Check sheet for the modelled part. Datum: model origin and axes. Units: mm. A direction names the side the tool comes from. Round coordinates to 2 decimals unless told otherwise and drop trailing zeros. Order: outer loops, then holes, each group sorted by start corner. A loop starts at its lowest first (then second) coordinate and runs counter-clockwise, first axis right, second up. Notation, with made-up numbers: (-1.75, 6) -> (52.25, 6) arc R18 ccw to (52.25, 38) -> close; hole circle Ø11 at (52, 8.5). An arc over 180 degrees is marked (long way). Answer in a Markdown table with one row per item.
from build123d import *

# Parameters (mm, degrees)
SKETCH1_R           = 4
SKETCH1_R_2         = 1.5
BOSS_EXTRUDE1_DEPTH = 4
SKETCH2_R           = 3.5
SKETCH2_R_2         = 2
CUT_EXTRUDE1_DEPTH  = 0.2
CUT_EXTRUDE2_START  = -0.2
SKETCH3_R           = 3.5
SKETCH3_R_2         = 2
CUT_EXTRUDE2_DEPTH  = 0.2


with BuildPart() as part:
    # Sketch1 → Boss-Extrude1 (new body)
    with BuildSketch(Plane(origin=(0, 0, 0), x_dir=(0, 0, -1), z_dir=(1, 0, 0))):
        Circle(SKETCH1_R)
        Circle(SKETCH1_R_2, mode=Mode.SUBTRACT)
    extrude(amount=BOSS_EXTRUDE1_DEPTH)

    # Sketch2 → Cut-Extrude1 (cut)
    with BuildSketch(Plane(origin=(4, 0, 0), x_dir=(0, 0, -1), z_dir=(1, 0, 0))):
        Circle(SKETCH2_R)
        Circle(SKETCH2_R_2, mode=Mode.SUBTRACT)
    extrude(amount=-CUT_EXTRUDE1_DEPTH, mode=Mode.SUBTRACT)

    # Sketch3 → Cut-Extrude2 (cut)
    with BuildSketch(Plane.ZY.offset(CUT_EXTRUDE2_START)):
        with Locations(Location((0, 0, 0), (0, 0, 180))):
            Circle(SKETCH3_R)
        with Locations(Location((0, 0, 0), (0, 0, 180))):
            Circle(SKETCH3_R_2, mode=Mode.SUBTRACT)
    extrude(amount=CUT_EXTRUDE2_DEPTH, mode=Mode.SUBTRACT)


solid = part.part
Item 1: Cross-section at D-D (x = 0.4). Record the boundary of the cut face in (y, z), and give its area (3 significant figures).
Result sheet:
| item | result |
|---|---|
| outline | circle Ø8 at (0, 0); hole circle Ø3 at (0, 0) |
| area | 43.2 mm^2 |
Item 2: Depth check by flat-ended pin: P1, Ø1.5, axis at x = 3, y = 1.5, coming from the +Z side; P2, Ø2, axis at x = 3.5, y = -2, coming from the -Z side; P3, Ø1.5, axis at x = 3.5, z = 2, coming from the +Y side. Enter the tip coordinate at first touch or a pass-through.
Result sheet:
| item | result |
|---|---|
| P1 | stops at z = 3.93 |
| P2 | stops at z = -3.87 |
| P3 | stops at y = 3.8 |
Item 3: Mould release check, pull along Y, two halves, no side actions. Record for faces 3 (the flat face through (3.8, -2, -2)), 4 (the cylindrical face through (1.972, -3.905, 0.867)): pulls with the +Y half, pulls with the -Y half, needs draft (parallel to the pull), parting line crosses it, or undercut.
Result sheet:
| item | result |
|---|---|
| face 3 | undercut |
| face 4 | parting line crosses it |
Item 4: Cross-section at A-A (z = 0). Record the boundary of the cut face in (x, y).
Result sheet:
| item | result |
|---|---|
| outline | (0, -4) -> (4, -4) -> (4, -3.5) -> (3.8, -3.5) -> (3.8, -2) -> (4, -2) -> (4, -1.5) -> (0, -1.5) -> (0, -2) -> (0.2, -2) -> (0.2, -3.5) -> (0, -3.5) -> close; (0, 1.5) -> (4, 1.5) -> (4, 2) -> (3.8, 2) -> (3.8, 3.5) -> (4, 3.5) -> (4, 4) -> (0, 4) -> (0, 3.5) -> (0.2, 3.5) -> (0.2, 2) -> (0, 2) -> close |
Item 5: Cross-section at C-C (z = -2.25). Record the boundary of the cut face in (x, y).
Result sheet:
| item | result |
|---|---|
| outline | (0, -3.31) -> (4, -3.31) -> (4, -2.68) -> (3.8, -2.68) -> (3.8, 2.68) -> (4, 2.68) -> (4, 3.31) -> (0, 3.31) -> (0, 2.68) -> (0.2, 2.68) -> (0.2, -2.68) -> (0, -2.68) -> close |
Item 6: Set-up check for faces 1 (the cylindrical face through (1.97, 0.07, 1.5)), 2 (the flat face through (0.2, 2, -2)): record each of +Z, -Z, +X, -X, +Y, -Y from which the full face is reachable in a straight line by a thin tool's end or side.
Result sheet:
| item | result |
|---|---|
| face 1 | +X, -X |
| face 2 | -X |
Item 7: Scan lines: line 1 (Y direction, x = 3.9, z = 0); line 2 (Y direction, x = 1.75, z = -1); line 3 (X direction, y = 2.5, z = -1.75). Record each from-to range of solid material in increasing order. Write a range as [from, to].
Result sheet:
| item | result |
|---|---|
| line 1 | y = [-4, -3.5], [-2, -1.5], [1.5, 2], [3.5, 4] |
| line 2 | y = [-3.87, -1.12], [1.12, 3.87] |
| line 3 | x = [0.2, 3.8] |
